Read the model definition and answer for the solid it produces. Units are mm, in the model's axes. Round coordinates to 2 decimals unless told otherwise and drop trailing zeros. Loops run counter-clockwise (first coordinate to the right, second up) from the corner with the lowest first, then second, coordinate; pieces in that order, holes last. Notation, with made-up numbers: (-36.5, 44.25) - (14.5, 44.25) arc R21 cw to (14.5, 66.25) - close; hole circle Ø4 at (-18.5, -0.75). An arc over 180 degrees is marked (long way). Use CSV: the item, a comma, the result in double quotes. Start each with the question number.
1. Find section A-A (x = 6.35). Give the vertices of the cut face in (y, z), and give its area (3 significant figures).
2. Find section B-B (x = 101.6). Give the vertices of the cut face in (y, z), and give its area (3 significant figures).
3. Consider line 1 along Y through (x, z) = (6.35, 0.7); line 2 along Y through (x, z) = (101.6, 1.55); line 3 along X through (y, z) = (171.45, 1.55). Determine where each line is inside the solid, lowest interval first.
4. Determine the mould class of faces 1 (the flat face through (100, 90, 0)), 2 (the cylindrical face through (199.49, 7.18, 1.31)) for opening direction Y: +Y half, -Y half, draft (parallel to the pull), parting line (faces both ways), or undercut.
from build123d import *

# Parameters (mm, degrees)
SKETCH1_W           = 203.2
SKETCH1_H           = 177.8
BOSS_EXTRUDE1_DEPTH = 2.667
SKETCH2_R           = 2.7686
CUT_EXTRUDE1_DEPTH  = 271.018875061


with BuildPart() as part:
    # Sketch1 → Boss-Extrude1 (new body)
    with BuildSketch(Plane.XY):
        with Locations((101.6, 88.9)):
            Rectangle(SKETCH1_W, SKETCH1_H)
    extrude(amount=BOSS_EXTRUDE1_DEPTH)

    # Sketch2 → Cut-Extrude1 (cut, through all)
    with BuildSketch(Plane.XY):
        with Locations((6.35, 6.35)):
            Circle(SKETCH2_R)
        with Locations((101.6, 6.35)):
            Circle(SKETCH2_R)
        with Locations((196.85, 6.35)):
            Circle(SKETCH2_R)
        with Locations((6.35, 88.9)):
            Circle(SKETCH2_R)
        with Locations((196.85, 88.9)):
            Circle(SKETCH2_R)
        with Locations((6.35, 171.45)):
            Circle(SKETCH2_R)
        with Locations((101.6, 171.45)):
            Circle(SKETCH2_R)
        with Locations((196.85, 171.45)):
            Circle(SKETCH2_R)
    extrude(amount=CUT_EXTRUDE1_DEPTH, mode=Mode.SUBTRACT)


solid = part.part
Filled sheet:
1,outline,"(0, 0) - (3.58, 0) - (3.58, 2.67) - (0, 2.67) - close; (9.12, 0) - (86.13, 0) - (86.13, 2.67) - (9.12, 2.67) - close; (91.67, 0) - (168.68, 0) - (168.68, 2.67) - (91.67, 2.67) - close; (174.22, 0) - (177.8, 0) - (177.8, 2.67) - (174.22, 2.67) - close"
1,area,"430 mm²"
2,outline,"(0, 0) - (3.58, 0) - (3.58, 2.67) - (0, 2.67) - close; (9.12, 0) - (168.68, 0) - (168.68, 2.67) - (9.12, 2.67) - close; (174.22, 0) - (177.8, 0) - (177.8, 2.67) - (174.22, 2.67) - close"
2,area,"445 mm²"
3,line 1,"y = 0 to 3.58, 9.12 to 86.13, 91.67 to 168.68, 174.22 to 177.8"
3,line 2,"y = 0 to 3.58, 9.12 to 168.68, 174.22 to 177.8"
3,line 3,"x = 0 to 3.58, 9.12 to 98.83, 104.37 to 194.08, 199.62 to 203.2"
4,face 1,"draft"
4,face 2,"undercut"
